from build123d import *

# Parameters (mm, degrees)
F1_DEPTH  = 50.8
F2_R      = 25.4
F3_R      = 38.1
F4_R      = 9.652
F5_DEPTH  = 241.3
F8_DEPTH  = 25.4
F10_DEPTH = 12.7
F12_DEPTH = 279.4
F13_R     = 5.08


with BuildPart() as f1:
    # F0 (on Front) → F1 (new body, symmetric)
    with BuildSketch(Plane.XZ):
        with BuildLine():
            ThreePointArc((-142.028809, -136.300183), (-182.631177, -73.455944), (-196.85, 0))
            Line((-196.85, 0), (-196.85, 25.4))
            Line((-196.85, 25.4), (-222.25, 25.4))
            Line((-222.25, 25.4), (-222.25, 0))
            ThreePointArc((-222.25, 0), (-204.061581, -88.056423), (-152.47332, -161.700183))
            Line((-152.47332, -161.700183), (-112.262965, -161.700183))
            Line((-112.262965, -161.700183), (112.262965, -161.700183))
            Line((112.262965, -161.700183), (152.47332, -161.700183))
            ThreePointArc((152.47332, -161.700183), (204.061581, -88.056423), (222.25, 0))
            Line((222.25, 0), (222.25, 25.4))
            Line((222.25, 25.4), (196.85, 25.4))
            Line((196.85, 25.4), (196.85, 0))
            ThreePointArc((196.85, 0), (182.631177, -73.455944), (142.028809, -136.300183))
            Line((142.028809, -136.300183), (-142.028809, -136.300183))
        make_face()
    extrude(amount=F1_DEPTH, both=True)

    # F2
    f2_edges = [f1.edges().sort_by_distance(p)[0] for p in [
        (-142.028809, 0, -136.300183),
        (-152.47332, 0, -161.700183),
        (152.47332, 0, -161.700183),
        (142.028809, 0, -136.300183),
    ]]
    fillet(f2_edges, radius=F2_R)

    # F3
    f3_edges = [f1.edges().sort_by_distance(p)[0] for p in [
        (-209.55, -50.8, 25.4),
        (-209.55, 50.8, 25.4),
        (209.55, 50.8, 25.4),
        (209.55, -50.8, 25.4),
    ]]
    fillet(f3_edges, radius=F3_R)

    # F4 (on Right) → F5 (cut, symmetric)
    with BuildSketch(Plane.YZ):
        Circle(F4_R)
    extrude(amount=F5_DEPTH, both=True, mode=Mode.SUBTRACT)

    # F7 (on Right) → F8 (join, symmetric)
    with BuildSketch(Plane.YZ):
        with BuildLine():
            Line((50.8, -153.887304), (50.8, -130.146238))
            ThreePointArc((50.8, -130.146238), (0, -114.202183), (-50.8, -130.146238))
            Line((-50.8, -130.146238), (-50.8, -153.887304))
            Line((-50.8, -153.887304), (-50.8, -161.700183))
            Line((-50.8, -161.700183), (50.8, -161.700183))
            Line((50.8, -161.700183), (50.8, -153.887304))
        make_face()
    extrude(amount=F8_DEPTH, both=True)

    # F9 (on Right) → F10 (cut, symmetric)
    with BuildSketch(Plane.YZ):
        with BuildLine():
            Line((50.8, -161.700183), (63.9712, -161.700183))
            ThreePointArc((63.9712, -161.700183), (0, -126.902183), (-63.9712, -161.700183))
            Line((-63.9712, -161.700183), (-50.8, -161.700183))
            Line((-50.8, -161.700183), (50.8, -161.700183))
        make_face()
    extrude(amount=F10_DEPTH, both=True, mode=Mode.SUBTRACT)

    # F11 (on Right) → F12 (cut, symmetric)
    with BuildSketch(Plane.YZ):
        with BuildLine():
            Line((-8.89, -110.49), (8.89, -110.49))
            ThreePointArc((8.89, -110.49), (22.360384, -104.910384), (27.94, -91.44))
            Line((27.94, -91.44), (27.94, -53.34))
            ThreePointArc((27.94, -53.34), (22.360384, -39.869616), (8.89, -34.29))
            Line((8.89, -34.29), (-8.89, -34.29))
            ThreePointArc((-8.89, -34.29), (-22.360384, -39.869616), (-27.94, -53.34))
            Line((-27.94, -53.34), (-27.94, -91.44))
            ThreePointArc((-27.94, -91.44), (-22.360384, -104.910384), (-8.89, -110.49))
        make_face()
    extrude(amount=F12_DEPTH, both=True, mode=Mode.SUBTRACT)

    # F13
    f13_edges = [f1.edges().sort_by_distance(p)[0] for p in [
        (12.7, 0, -126.902183),
        (-12.7, 0, -126.902183),
    ]]
    fillet(f13_edges, radius=F13_R)


solid = f1.part
Geometry check sheet. Reference: the model listing, model coordinates, mm. A direction names the side the tool comes from. Give positions to 0.01 mm unless a question says otherwise; leave off trailing zeros. Order: outer loops, then holes, each group sorted by start corner. A loop starts at its lowest first (then second) coordinate and runs counter-clockwise, first axis right, second up.
1. Scan lines: line 1 (Z direction, x = 217.25, y = 0); line 2 (X direction, y = -12.5, z = -118.5); line 3 (X direction, y = 3.5, z = 17). Record each from-to range of solid material in increasing order.
Completed:
line 1: z = -34.29 to -9.65, 9.65 to 25.4
line 2: x = -188.02 to -157.19, -25.4 to 25.4, 157.19 to 188.02
line 3: x = -222.25 to -196.85, 196.85 to 222.25
2. Sectioned sample at C-C (x = 82). Record the boundary of the cut face in (y, z), then the cut area to 3 significant figures.
Completed:
outline: (-50.8, -161.7) - (50.8, -161.7) - (50.8, -136.3) - (-50.8, -136.3) - close
area: 2,580 mm2
3. Access from +Z, -Z, +X, -X, +Y, -Y to the whole of each face (thin tool, end or side, straight path). Record for faces 1 (the face through (183.02, -22.51, -104.76)), 2 (the face through (141.29, 0.71, -134.01)), 3 (the face through (0.356, 0.757, -114.205)), 4 (the face through (-207, 0, -34.29)), 5 (the face through (-178, 0, -110.49)).
Completed:
face 1: +X, -X
face 2: +Z, +Y, -Y
face 3: +Z
face 4: -Z, +X, -X
face 5: +Z, +X, -X
4. Sectioned sample at B-B (y = 0). State how many separate pieces and enclosed holes the cut face has, then the cut area to 3 significant figures.
Completed:
separate pieces: 5
enclosed holes: 0
area: 12,300 mm2
5. Depth check by flat-ended pin: pin 1 (6.5 mm diameter, centred on y = -17, z = -122, fed in from -X); pin 2 (1.5 mm diameter, centred on y = -10, z = -138.5, fed in from -X); pin 3 (19.5 mm diameter, centred on x = -206, y = -2.5, fed in from -Z). Enter the tip coordinate at first touch or a pass-through.
Completed:
pin 1: stops at x = -187.87
pin 2: stops at x = -174.41
pin 3: stops at z = -34.59
6. Draft check along Z on faces 6 (the face through (222.25, -1, 13)), 7 (the face through (-141.57, 0.71, -133.88)), 8 (the face through (-182.46, -22.51, -104.76)). Enter one of: pulls with the +Z half, pulls with the -Z half, needs draft (parallel to the pull), parting line crosses it, or undercut.
Completed:
face 6: needs draft
face 7: pulls with the +Z half
face 8: undercut
7. Sectioned sample at A-A (z = -70.5). Record the boundary of the cut face in (x, y), then the cut area to 3 significant figures.
Completed:
outline: (-210.77, -50.8) - (-183.79, -50.8) - (-183.79, -27.94) - (-210.77, -27.94) - close; (-210.77, 27.94) - (-183.79, 27.94) - (-183.79, 50.8) - (-210.77, 50.8) - close; (183.79, -50.8) - (210.77, -50.8) - (210.77, -27.94) - (183.79, -27.94) - close; (183.79, 27.94) - (210.77, 27.94) - (210.77, 50.8) - (183.79, 50.8) - close
area: 2,470 mm2
